from build123d import *

# Parameters (mm, degrees)
F0_R     = 7.5
F1_DEPTH = 2.5
F2_R     = 3.25
F3_DEPTH = 7.4
F4_W     = 1.5
F4_H     = 16
F5_DEPTH = 1.5
F7_D     = 3.3


with BuildPart() as f1:
    # F0 (on Top) → F1 (new body)
    with BuildSketch(Plane.XY):
        Circle(F0_R)
    extrude(amount=F1_DEPTH)

    # F2 (on face) → F3 (join)
    with BuildSketch(Plane.XY.offset(2.5)):
        Circle(F2_R)
    extrude(amount=F3_DEPTH)

    # F4 (on face) → F5 (cut)
    with BuildSketch(Plane(origin=(0, 0, 0), x_dir=(1, 0, 0), z_dir=(0, 0, -1))):
        Rectangle(F4_W, F4_H)
    extrude(amount=-F5_DEPTH, mode=Mode.SUBTRACT)

    # F7 (through all)
    with Locations(Plane.XY.offset(9.9)):
        with Locations((0, 0)):
            Hole(F7_D / 2)


solid = f1.part
CAD build for the part. Positions are in the model's coordinates, mm. A direction names the side the tool comes from. Round coordinates to 2 decimals unless told otherwise and drop trailing zeros. Write each loop counter-clockwise with the first axis right and the second up, starting at its lowest first coordinate (ties: lowest second). Pieces come first, ordered by that corner, then holes.
(1) Slice it at B-B, the plane x = 0. Write the cut outline in (y, z).
(2) Slice it at D-D, the plane z = 7. Write the cut outline in (x, y).
(3) Drop flat-ended pins along their axis: P1, Ø1.2, axis at y = -3.5, z = 0.5, coming from the -X side; P2, Ø1, axis at y = 5.5, z = 6, coming from the -X side; P3, Ø1.6, axis at y = -4, z = 0.5, coming from the +X side; P4, Ø0.8, axis at x = 0, y = 3.5, coming from the -Z side. Give the stop position or say it passes through.
(4) Probe line 1 along Y through (x, z) = (0, 7); line 2 along Z through (x, y) = (5.75, 4.75); line 3 along Y through (x, z) = (1.75, 5.25). List the from-to ranges inside material, lowest first.
(5) 3-axis set-ups, long thin cutter, end or side, ignore diameter. For faces 1 (the face through (0, -5, 1.5)), 2 (the face through (-2.579, -1.978, 6.148)), 3 (the face through (-3, 0, 0)): which of +Z, -Z, +X, -X, +Y, -Y reach the whole face in a straight line?
(6) Mould opens along Y. For faces 4 (the face through (3, 0, 0)), 5 (the face through (-1.524, -0.632, 4.881)), 6 (the face through (-7.493, 0.33, 1.232)) say: pulls with the +Y half, pulls with the -Y half, needs draft (parallel to the pull), parting line crosses it, or undercut.
(7) Slice it at A-A, the plane y = 0. Write the cut outline in (x, z), and give its area (3 significant figures).
(8) Slice it at C-C, the plane y = 5.75. Write the cut outline in (x, z).
From the geometry:
1. outline: (-7.5, 1.5) - (-1.65, 1.5) - (-1.65, 9.9) - (-3.25, 9.9) - (-3.25, 2.5) - (-7.5, 2.5) - close; (1.65, 1.5) - (7.5, 1.5) - (7.5, 2.5) - (3.25, 2.5) - (3.25, 9.9) - (1.65, 9.9) - close
2. outline: circle Ø6.5 at (0, 0); hole circle Ø3.3 at (0, 0)
3. P1: stops at x = -6.92
3. P2: passes through
3. P3: stops at x = 6.78
3. P4: stops at z = 1.5
4. line 1: y = -3.25 to -1.65, 1.65 to 3.25
4. line 2: z = 0 to 2.5
4. line 3: y = -2.74 to 2.74
5. face 1: -Z, +Y, -Y
5. face 2: +Z
5. face 3: -Z, +X, -X, +Y, -Y
6. face 4: needs draft
6. face 5: undercut
6. face 6: parting line crosses it
7. outline: (-7.5, 0) - (-1.65, 0) - (-1.65, 9.9) - (-3.25, 9.9) - (-3.25, 2.5) - (-7.5, 2.5) - close; (1.65, 0) - (7.5, 0) - (7.5, 2.5) - (3.25, 2.5) - (3.25, 9.9) - (1.65, 9.9) - close
7. area: 52.9 mm2
8. outline: (-4.82, 0) - (-0.75, 0) - (-0.75, 1.5) - (0.75, 1.5) - (0.75, 0) - (4.82, 0) - (4.82, 2.5) - (-4.82, 2.5) - close
